```python
from build123d import *

# Parameters (mm, degrees)
PAD_DEPTH       = 5
POCKET_DEPTH    = 5
SKETCH002_R     = 1.6
POCKET001_DEPTH = 5
SKETCH003_R     = 3
POCKET002_DEPTH = 3
SKETCH004_R     = 6.15
POCKET003_DEPTH = 5
POCKET004_DEPTH = 2
SKETCH006_R     = 0.95
POCKET005_DEPTH = 3
FILLET_R        = 1


with BuildPart() as part:
    # Sketch → Pad (new body)
    with BuildSketch(Plane.XY):
        with BuildLine():
            Line((-35, 70), (35, 70))
            ThreePointArc((55, 50), (49.142136, 64.142136), (35, 70))
            Line((55, 50), (55, 25))
            ThreePointArc((30, 0), (47.67767, 7.32233), (55, 25))
            Line((30, 0), (-30, 0))
            ThreePointArc((-55, 25), (-47.67767, 7.32233), (-30, 0))
            Line((-55, 25), (-55, 50))
            ThreePointArc((-35, 70), (-49.142136, 64.142136), (-55, 50))
        make_face()
    extrude(amount=PAD_DEPTH)

    # Sketch001 (on Face10 of Pad) → Pocket (cut)
    with BuildSketch(Plane.XY.offset(5)):
        with BuildLine():
            Line((-10, 58), (10, 58))
            ThreePointArc((20, 48), (17.071068, 55.071068), (10, 58))
            Line((20, 48), (20, 22))
            ThreePointArc((10, 12), (17.071068, 14.928932), (20, 22))
            Line((10, 12), (-10, 12))
            ThreePointArc((-20, 22), (-17.071068, 14.928932), (-10, 12))
            Line((-20, 22), (-20, 48))
            ThreePointArc((-10, 58), (-17.071068, 55.071068), (-20, 48))
        make_face()
    extrude(amount=-POCKET_DEPTH, mode=Mode.SUBTRACT)

    # Sketch002 (on Face5 of Pocket) → Pocket001 (cut)
    with BuildSketch(Plane.XY.offset(5)):
        with Locations((-5, 6)):
            Circle(SKETCH002_R)
        with Locations((5, 6)):
            Circle(SKETCH002_R)
        with Locations((15, 64)):
            Circle(SKETCH002_R)
        with Locations((-15, 64)):
            Circle(SKETCH002_R)
    extrude(amount=-POCKET001_DEPTH, mode=Mode.SUBTRACT)

    # Sketch003 (on Face5 of Pocket001) → Pocket002 (cut)
    with BuildSketch(Plane.XY.offset(5)):
        with Locations((-15, 64)):
            Circle(SKETCH003_R)
        with Locations((15, 64)):
            Circle(SKETCH003_R)
        with Locations((-5, 6)):
            Circle(SKETCH003_R)
        with Locations((5, 6)):
            Circle(SKETCH003_R)
    extrude(amount=-POCKET002_DEPTH, mode=Mode.SUBTRACT)

    # Sketch004 (on Face5 of Pocket002) → Pocket003 (cut)
    with BuildSketch(Plane.XY.offset(5)):
        with Locations((-39, 44)):
            Circle(SKETCH004_R)
        with Locations((39, 44)):
            Circle(SKETCH004_R)
    extrude(amount=-POCKET003_DEPTH, mode=Mode.SUBTRACT)

    # Sketch005 (on Face5 of Pocket003) → Pocket004 (cut)
    with BuildSketch(Plane.XY.offset(5)):
        with BuildLine():
            ThreePointArc((-36.432447, 57.909479), (-39, 60.1), (-41.567553, 57.909479))
            Line((-41.567553, 57.909479), (-42.75, 50.495191))
            Line((-49.762186, 53.178305), (-42.75, 50.495191))
            ThreePointArc((-49.762186, 53.178305), (-52.943009, 52.05), (-52.329739, 48.731174))
            Line((-46.5, 44), (-52.329739, 48.731174))
            Line((-52.329739, 39.268826), (-46.5, 44))
            ThreePointArc((-52.329739, 39.268826), (-52.943009, 35.95), (-49.762186, 34.821695))
            Line((-42.75, 37.504809), (-49.762186, 34.821695))
            Line((-41.567553, 30.090521), (-42.75, 37.504809))
            ThreePointArc((-41.567553, 30.090521), (-39, 27.9), (-36.432447, 30.090521))
            Line((-35.25, 37.504809), (-36.432447, 30.090521))
            Line((-28.237814, 34.821695), (-35.25, 37.504809))
            ThreePointArc((-28.237814, 34.821695), (-25.056991, 35.95), (-25.670261, 39.268826))
            Line((-31.5, 44), (-25.670261, 39.268826))
            Line((-25.670261, 48.731174), (-31.5, 44))
            ThreePointArc((-25.670261, 48.731174), (-25.056991, 52.05), (-28.237814, 53.178305))
            Line((-35.25, 50.495191), (-28.237814, 53.178305))
            Line((-36.432447, 57.909479), (-35.25, 50.495191))
        make_face()
        with BuildLine():
            ThreePointArc((41.567553, 57.909479), (39, 60.1), (36.432447, 57.909479))
            Line((36.432447, 57.909479), (35.25, 50.495191))
            Line((35.25, 50.495191), (28.237814, 53.178305))
            ThreePointArc((28.237814, 53.178305), (25.056991, 52.05), (25.670261, 48.731174))
            Line((25.670261, 48.731174), (31.5, 44))
            Line((31.5, 44), (25.670261, 39.268826))
            ThreePointArc((25.670261, 39.268826), (25.056991, 35.95), (28.237814, 34.821695))
            Line((28.237814, 34.821695), (35.25, 37.504809))
            Line((35.25, 37.504809), (36.432447, 30.090521))
            ThreePointArc((36.432447, 30.090521), (39, 27.9), (41.567553, 30.090521))
            Line((41.567553, 30.090521), (42.75, 37.504809))
            Line((42.75, 37.504809), (49.762186, 34.821695))
            ThreePointArc((49.762186, 34.821695), (52.943009, 35.95), (52.329739, 39.268826))
            Line((52.329739, 39.268826), (46.5, 44))
            Line((46.5, 44), (52.329739, 48.731174))
            ThreePointArc((52.329739, 48.731174), (52.943009, 52.05), (49.762186, 53.178305))
            Line((49.762186, 53.178305), (42.75, 50.495191))
            Line((42.75, 50.495191), (41.567553, 57.909479))
        make_face()
    extrude(amount=-POCKET004_DEPTH, mode=Mode.SUBTRACT)

    # Sketch006 (on Face68 of Pocket004) → Pocket005 (cut)
    with BuildSketch(Plane.XY.offset(3)):
        with Locations((-39, 54.5)):
            Circle(SKETCH006_R)
        with Locations((-29.906733, 49.25)):
            Circle(SKETCH006_R)
        with Locations((-29.906733, 38.75)):
            Circle(SKETCH006_R)
        with Locations((-39, 33.5)):
            Circle(SKETCH006_R)
        with Locations((-48.093267, 38.75)):
            Circle(SKETCH006_R)
        with Locations((-48.093267, 49.25)):
            Circle(SKETCH006_R)
        with Locations((29.906733, 49.25)):
            Circle(SKETCH006_R)
        with Locations((39, 54.5)):
            Circle(SKETCH006_R)
        with Locations((48.093267, 49.25)):
            Circle(SKETCH006_R)
        with Locations((48.093267, 38.75)):
            Circle(SKETCH006_R)
        with Locations((39, 33.5)):
            Circle(SKETCH006_R)
        with Locations((29.906733, 38.75)):
            Circle(SKETCH006_R)
    extrude(amount=-POCKET005_DEPTH, mode=Mode.SUBTRACT)

    # Fillet
    fillet_edges = [part.edges().sort_by_distance(p)[0] for p in [
        (-42.75, 50.495191, 4),
        (-35.25, 50.495191, 4),
        (-31.5, 44, 4),
        (-46.5, 44, 4),
        (35.25, 50.495191, 4),
        (42.75, 50.495191, 4),
        (31.5, 44, 4),
        (46.5, 44, 4),
        (-42.75, 37.504809, 4),
        (-35.25, 37.504809, 4),
        (35.25, 37.504809, 4),
        (42.75, 37.504809, 4),
    ]]
    fillet(fillet_edges, radius=FILLET_R)


solid = part.part
```
Work out the finished part from the listing and answer in its coordinate system (mm). A direction names the side the tool comes from. Give positions to 0.01 mm unless a question says otherwise; leave off trailing zeros. Write each loop counter-clockwise with the first axis right and the second up, starting at its lowest first coordinate (ties: lowest second). Pieces come first, ordered by that corner, then holes. Notation, with made-up numbers: (69, 59) - (95, 59) arc R20 cw to (95, 87) - close; hole circle Ø8 at (64.25, 44). An arc over 180 degrees is marked (long way). Use one line per item in the form item = value.
1. A cutting plane is placed at B-B (y = 64). Write down the section's boundary in (x, z).
Filled in:
outline = (-49.28, 0) - (-16.6, 0) - (-16.6, 2) - (-18, 2) - (-18, 5) - (-49.28, 5) - close; (-13.4, 0) - (13.4, 0) - (13.4, 2) - (12, 2) - (12, 5) - (-12, 5) - (-12, 2) - (-13.4, 2) - close; (16.6, 0) - (49.28, 0) - (49.28, 5) - (18, 5) - (18, 2) - (16.6, 2) - close
2. For faces 1 (the face through (-16.99, 55.15, 2.54)), 2 (the face through (-42.055, 54.854, 4.014)), 3 (the face through (49.297, 63.986, 2.465)), determine the directions among +Z, -Z, +X, -X, +Y, -Y from which every point of the face is accessible in a straight line to the end or side of a thin tool.
Filled in:
face_1 = +Z, -Z
face_2 = +Z
face_3 = +Z, -Z, +X, +Y
3. Consider L1, parallel to Y at x = 5, z = 3.2; L2, parallel to X at y = 33.5, z = 1.05; L3, parallel to Y at x = 17.5, z = 2.5. Determine where each line is inside the solid, lowest interval first.
Filled in:
L1 = 0 to 3, 9 to 12, 58 to 70
L2 = -55 to -39.95, -38.05 to -20, 20 to 38.05, 39.95 to 55
L3 = 0 to 15.39, 54.61 to 62.34, 65.66 to 70
4. A cutting plane is placed at D-D (y = 46). Write down the section's boundary in (x, z), and give its area (3 significant figures).
Filled in:
outline = (-55, 0) - (-44.82, 0) - (-44.82, 3) - (-48.96, 3) - (-48.96, 5) - (-55, 5) - close; (-33.18, 0) - (-20, 0) - (-20, 5) - (-29.04, 5) - (-29.04, 3) - (-33.18, 3) - close; (20, 0) - (33.18, 0) - (33.18, 3) - (29.04, 3) - (29.04, 5) - (20, 5) - close; (44.82, 0) - (55, 0) - (55, 5) - (48.96, 5) - (48.96, 3) - (44.82, 3) - close
area = 200 mm^2
5. A cutting plane is placed at C-C (z = 1.05). State how many separate pieces and enclosed holes the cut face has, and give its area (3 significant figures).
Filled in:
separate_pieces = 1
enclosed_holes = 19
area = 5,200 mm^2
6. A cutting plane is placed at A-A (x = -5). Write down the section's boundary in (y, z), and give its area (3 significant figures).
Filled in:
outline = (0, 0) - (4.4, 0) - (4.4, 2) - (3, 2) - (3, 5) - (0, 5) - close; (7.6, 0) - (12, 0) - (12, 5) - (9, 5) - (9, 2) - (7.6, 2) - close; (58, 0) - (70, 0) - (70, 5) - (58, 5) - close
area = 95.6 mm^2
7. Each of these flat-tipped pins is pushed along its axis until it touches: pin 1 Ø2 at (x, y) = (29.91, 49.25) entering from +Z; pin 2 Ø5 at (x, y) = (-15, 64) entering from +Z. Where does it stop, or does it pass through?
Filled in:
pin_1 = 3
pin_2 = 2
8. Determine the mould class of faces 4 (the face through (-13.7, 62.7, 2)), 5 (the face through (47.482, 7.129, 2.465)), 6 (the face through (-24, 35, 5)) for opening direction Y: released by +Y, released by -Y, zero draft, split by the parting line, or undercut.
Filled in:
face_4 = undercut
face_5 = released by -Y
face_6 = zero draft
